Could you check a few things on this model? Use its own coordinates, in mm. Give positions to 0.01 mm unless a question says otherwise; leave off trailing zeros. Write each loop counter-clockwise with the first axis right and the second up, starting at its lowest first coordinate (ties: lowest second). Pieces come first, ordered by that corner, then holes. Notation, with made-up numbers: (36, 58.25) - (61, 58.25) arc R12 cw to (61, 73.25) - close; hole circle Ø2 at (-15.75, 37). An arc over 180 degrees is marked (long way). Answer in a Markdown table with one row per item.
from build123d import *

# Parameters (mm, degrees)
ESTRUSIONE_ESTRUSIONE1_START = 17
SCHIZZO1_W                   = 115
SCHIZZO1_H                   = 60
ESTRUSIONE_ESTRUSIONE1_DEPTH = 2
SCHIZZO5_R                   = 1.5
ESTRUSIONE_ESTRUSIONE2_DEPTH = 19
SCHIZZO6_R                   = 1.5
ESTRUSIONE_ESTRUSIONE3_DEPTH = 19
SCHIZZO1_3_W                 = 115
SCHIZZO1_3_H                 = 60
ESTRUSIONE_ESTRUSIONE4_DEPTH = 1


with BuildPart() as part:
    # Schizzo1 → Estrusione-Estrusione1 (new body)
    with BuildSketch(Plane(origin=(0, 2, 0), x_dir=(1, 0, 0), z_dir=(0, 1, 0)).offset(ESTRUSIONE_ESTRUSIONE1_START)):
        with Locations((-164.562548693, 37.708245302)):
            Rectangle(SCHIZZO1_W, SCHIZZO1_H)
    extrude(amount=ESTRUSIONE_ESTRUSIONE1_DEPTH)

    # Schizzo5 → Estrusione-Estrusione2 (add)
    with BuildSketch(Plane(origin=(0, 21, 0), x_dir=(1, 0, 0), z_dir=(0, 1, 0))):
        with Locations((-111.062548693, 63.708245302)):
            Circle(SCHIZZO5_R)
    extrude(amount=-ESTRUSIONE_ESTRUSIONE2_DEPTH)

    # Schizzo6 → Estrusione-Estrusione3 (add)
    with BuildSketch(Plane(origin=(0, 21, 0), x_dir=(1, 0, 0), z_dir=(0, 1, 0))):
        with Locations((-192.062548693, 63.708245302)):
            Circle(SCHIZZO6_R)
    extrude(amount=-ESTRUSIONE_ESTRUSIONE3_DEPTH)

    # Schizzo1<3> → Estrusione-Estrusione4 (add)
    with BuildSketch(Plane(origin=(0, 2, 0), x_dir=(1, 0, 0), z_dir=(0, 1, 0))):
        with Locations((-164.562548693, 37.708245302)):
            Rectangle(SCHIZZO1_3_W, SCHIZZO1_3_H)
    extrude(amount=ESTRUSIONE_ESTRUSIONE4_DEPTH)


solid = part.part
1) We'd pull the mould along Y, two halves only. Please class faces 1 (the face through (-112.56, 11.11, -63.77)), 2 (the face through (-190.68, 11.11, -63.13)), 3 (the face through (-165, 2, -38)), 4 (the face through (-222.063, 20, -37)): +Y half, -Y half, draft (parallel to the pull), parting line (faces both ways), or undercut.
Check values:
| item | result |
|---|---|
| face 1 | undercut |
| face 2 | undercut |
| face 3 | -Y half |
| face 4 | draft |
2) Imagine slicing it at B-B (x = -139). List the corners of the cut face in (y, z) for me, then the cut area to 3 significant figures.
Check values:
| item | result |
|---|---|
| outline | (2, -67.71) - (3, -67.71) - (3, -7.71) - (2, -7.71) - close; (19, -67.71) - (21, -67.71) - (21, -7.71) - (19, -7.71) - close |
| area | 180 mm2 |
3) If I drill on line 1 (Y direction, x = -151.5, z = -19); line 2 (X direction, y = 6.75, z = -62.5); line 3 (X direction, y = 17, z = -64), over which ranges is the centre line in solid material (lowest first)?
Check values:
| item | result |
|---|---|
| line 1 | y = 2 to 3, 19 to 21 |
| line 2 | x = -192.95 to -191.17, -111.95 to -110.17 |
| line 3 | x = -193.53 to -190.59, -112.53 to -109.59 |
4) Imagine slicing it at C-C (x = -192). List the corners of the cut face in (y, z) for me.
Check values:
| item | result |
|---|---|
| outline | (2, -67.71) - (3, -67.71) - (3, -65.21) - (19, -65.21) - (19, -67.71) - (21, -67.71) - (21, -7.71) - (19, -7.71) - (19, -62.21) - (3, -62.21) - (3, -7.71) - (2, -7.71) - close |
5) Imagine slicing it at A-A (z = -18.5). List the corners of the cut face in (x, y) for me, then the cut area to 3 significant figures.
Check values:
| item | result |
|---|---|
| outline | (-222.06, 2) - (-107.06, 2) - (-107.06, 3) - (-222.06, 3) - close; (-222.06, 19) - (-107.06, 19) - (-107.06, 21) - (-222.06, 21) - close |
| area | 345 mm2 |
6) Imagine slicing it at D-D (y = 5.25). List the corners of the cut face in (x, z) for me.
Check values:
| item | result |
|---|---|
| outline | circle Ø3 at (-192.06, -63.71); circle Ø3 at (-111.06, -63.71) |
